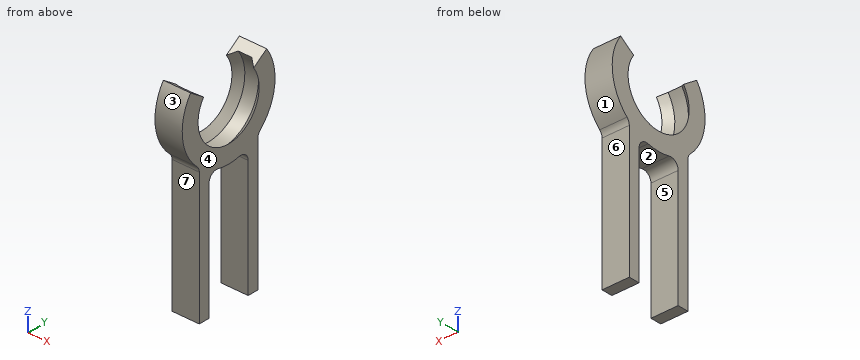
Autodesk Inventor part; units mm, degrees
ref_plane "YZ Plane" through (0, 0, 0) normal (1, 0, 0) x (0, 1, 0)
ref_plane "XZ Plane" through (0, 0, 0) normal (0, 1, 0) x (-1, 0, 0)
ref_plane "XY Plane" through (0, 0, 0) normal (0, 0, 1) x (1, 0, 0)
sketch "Sketch4" plane through (0, 0, 0) normal (0, 1, 0) x (-1, 0, 0)
  line L0 (1, -2.5) -> (1, -3.8)
  line L1 (1, -3.8) -> (-1, -3.8)
  line L2 (-1, -3.8) -> (-1, -2.5)
  line L3 (-1, -2.5) -> (-0.5, -3)
  line L4 (-0.5, -3) -> (0.5, -3)
  line L5 (0.5, -3) -> (1, -2.5)
  line L6 (0, 0) -> (-1.4783, 0)
  point P0 (0, -3)
  dimension "d21" = 1
  dimension "d22" = 3
  dimension "d24" = 0.8
  dimension "d32" = 0.5
revolve "Revolution1" add sketch "Sketch4" angle 250 mid plane about axis through (0, 0, 0) along (1, 0, 0)
sketch "Sketch5" plane through (1, 0, 0) normal (1, 0, 0) x (0, 0, -1)
  arc A0 (-2.1796, -3.1128) -> (-2.1796, 3.1128) centre (0, 0) ccw
  line L0 (2.9462, -2.4) -> (12.9462, -2.4)
  line L1 (12.9462, -2.4) -> (12.9462, -1.6)
  line L2 (12.9462, -1.6) -> (3.4467, -1.6)
  line L3 (3.4467, 1.6) -> (12.9462, 1.6)
  line L4 (12.9462, 1.6) -> (12.9462, 2.4)
  line L5 (12.9462, 2.4) -> (2.9462, 2.4)
  point P0 (0, 0)
  point P1 (12.9462, 2)
  point P2 (12.9462, -2)
  dimension "d26" = 0.8
  dimension "d27" = 10
  dimension "d28" = 4
  dimension "d10" = 1.5
  dimension "d11" = 0.8
  dimension "d12" = 6
  dimension "d13" = 5.5
  dimension "d14" = 0.5
  dimension "d15" = 0.8
  dimension "d16" = 8
extrude "Extrusion5" add sketch "Sketch5" against normal up to surface (2 mm away)
fillet "Fillet1" radius 0.6 4 edges at (0, 2.4, -2.9462) (0, 1.6, -3.4467) (0, -1.6, -3.4467) (0, -2.4, -2.9462)
sketch "Sketch1" plane through (0, 0, 0) normal (0, 1, 0) x (-1, 0, 0)
  line L0 (-1, 2.3) -> (0, 3.3)
  line L1 (0, 3.3) -> (1, 2.3)
  line L2 (1, 2.3) -> (1, 4.5)
  line L3 (1, 4.5) -> (-1, 4.5)
  line L4 (-1, 4.5) -> (-1, 2.3)
  line L5 (0, 0) -> (-2.1371, 0)
  line L6 (-1, -2.3) -> (0, -3.3)
  line L7 (0, -3.3) -> (1, -2.3)
  line L8 (1, -2.3) -> (1, -4.5)
  line L9 (1, -4.5) -> (-1, -4.5)
  line L10 (-1, -4.5) -> (-1, -2.3)
  dimension "d0" = 45
  dimension "d1" = 3.3
  dimension "d2" = 2
  dimension "d3" = 4.5
sketch "Sketch2" plane through (-1, 0, 4.5) normal (0, 0, 1) x (1, 0, 0)
  line L0 (0, 0) -> (2, 0)
  line L1 (2, 0) -> (2, -2)
  line L2 (2, -2) -> (-3, -2)
  line L3 (-3, -2) -> (0, 0)
  point P0 (1, 0)
  dimension "d6" = 2
  dimension "d7" = 5
properties part number "6mm lens mount"
Geometry: final body of the model. Coordinates: model frame, mm. Face numbers are marked on the shaded views. A direction names the side the tool comes from. Give positions to 0.01 mm unless a question says otherwise; leave off trailing zeros. Loops run counter-clockwise (first coordinate to the right, second up) from the corner with the lowest first, then second, coordinate; pieces in that order, holes last. Notation, with made-up numbers: (-12, 30.25) - (24, 30.25) arc R28 ccw to (24, 65.25) - close; hole circle Ø9 at (44, 45.5). An arc over 180 degrees is marked (long way). Answer as CSV lines item,"result". Start each with the question number.
1. Ray query, L1, parallel to Y at x = -0.2, z = -6; L2, parallel to Y at x = 0, z = 0; L3, parallel to Z at x = -0.3, y = 1.25. Return the intervals inside material, ascending.
2. Section A-A, the plane z = 0. Return loops of the section in (x, y), plus the area to 3 significant figures.
3. Section B-B, the plane z = -8. Return loops of the section in (x, y), plus the area to 3 significant figures.
4. Draft query along Y for the marked faces 1, 2 and 3. Return one class per face: released by +Y, released by -Y, zero draft, split by the parting line, or undercut.
5. Section D-D, the plane x = 0.8. Return loops of the section in (y, z), plus the area to 3 significant figures.
6. Section C-C, the plane y = 0. Return loops of the section in (x, z), plus the area to 3 significant figures.
7. Pin query (flat end, axial travel): P1, Ø1, axis at x = 0, z = -7, coming from the -Y side. Return the tip coordinate at first contact, or that it passes through.
8. Reachability of the marked faces 4, 5, 6 and 7 from +Z, -Z, +X, -X, +Y, -Y: full face, straight path, thin tool, end or side. Return the list, or none.
Answers:
1,L1,"y = -2.4 to -1.6, 1.6 to 2.4"
1,L2,"y = -3.8 to -3, 3 to 3.8"
1,L3,"z = -3.74 to -2.73"
2,outline,"(-1, -3.8) - (1, -3.8) - (1, -2.5) - (0.5, -3) - (-0.5, -3) - (-1, -2.5) - close; (-1, 2.5) - (-0.5, 3) - (0.5, 3) - (1, 2.5) - (1, 3.8) - (-1, 3.8) - close"
2,area,"3.70 mm2"
3,outline,"(-1, -2.4) - (1, -2.4) - (1, -1.6) - (-1, -1.6) - close; (-1, 1.6) - (1, 1.6) - (1, 2.4) - (-1, 2.4) - close"
3,area,"3.20 mm2"
4,face 1,"released by +Y"
4,face 2,"undercut"
4,face 3,"released by -Y"
5,outline,"(-3.11, 2.18) arc R3.8 ccw to (-2.59, -2.78) arc R0.6 cw to (-2.4, -3.22) - (-2.4, -12.95) - (-1.6, -12.95) - (-1.6, -4.28) arc R0.6 cw to (-0.86, -3.7) arc R3.8 ccw to (0.86, -3.7) arc R0.6 cw to (1.6, -4.28) - (1.6, -12.95) - (2.4, -12.95) - (2.4, -3.22) arc R0.6 cw to (2.59, -2.78) arc R3.8 ccw to (3.11, 2.18) - (2.21, 1.55) arc R2.7 cw (long way) to (-2.21, 1.55) - close"
5,area,"31.5 mm2"
6,outline,"(-1, -3.8) - (1, -3.8) - (1, -2.5) - (0.5, -3) - (-0.5, -3) - (-1, -2.5) - close"
6,area,"1.85 mm2"
7,P1,"stops at y = -2.4"
8,face 4,"+Z, -Z, +X, +Y, -Y"
8,face 5,"-Z, +X, -X"
8,face 6,"-Z, +X, -X, +Y"
8,face 7,"-Z, +X, -X, -Y"
